The model under review builds one solid part; all positions refer to its coordinate system, in mm. Face numbers are marked on the shaded views. A direction names the side the tool comes from. Coordinates: 2 decimals unless noted, no trailing zeros. Loops run counter-clockwise (first coordinate to the right, second up) from the corner with the lowest first, then second, coordinate; pieces in that order, holes last. Notation, with made-up numbers: (70, 61.5) - (84, 61.5) arc R24 cw to (84, 84.5) - close; hole circle Ø4 at (-37.75, 63.25). An arc over 180 degrees is marked (long way). One line per item, written item: value. Start each with the question number.
1. We need section A-A, the plane x = 0. Give the boundary of the cut face in (y, z).
2. Mouldability with a two-part tool opening along X and no side actions: class the marked faces 4, 5 and 6 as +X half, -X half, draft (parallel to the pull), parting line (faces both ways), or undercut.
3. We need section D-D, the plane y = 0. Give the boundary of the cut face in (x, z).
4. To check wall thickness, follow line 1 (Y direction, x = 0.5, z = -23); line 2 (Z direction, x = -26, y = -8); line 3 (Z direction, x = -22, y = -14.5). State the ranges of each line that lie inside material, in increasing order.
5. Insertion check: P1, Ø13, axis at x = -20.12, z = 9.25, coming from the +Y side; P2, Ø4, axis at x = -20.12, z = 9.25, coming from the -Y side; P3, Ø0.6, axis at y = -17.5, z = 0, coming from the -X side; P4, Ø3, axis at x = -23.5, z = -13.5, coming from the -Y side. Each pin has a flat end and moves straight along its axis. Give the tip position at first contact, or say it passes through.
6. We need section B-B, the plane z = -24.25. Give the boundary of the cut face in (x, y).
7. We need section C-C, the plane x = -14. Give the boundary of the cut face in (y, z).
8. For the marked faces 1, 2 and 3, list the 3-axis set-ups (+Z, -Z, +X, -X, +Y, -Y) from which the entire face can be reached by the end or side of a thin tool; tool diameter is ignored.
from build123d import *

# Parameters (mm, degrees)
F1_DEPTH       = 35
F3_D           = 5
F3_START       = 1.7550021
F3_CBORE_D     = 10
F3_CBORE_DEPTH = 8
F4_W           = 22.4
F4_H           = 2
F5_DEPTH       = 25
F6_R           = 6
F7_DEPTH       = 8


with BuildPart() as f1:
    # F0 (on Top) → F1 (new body, symmetric)
    with BuildSketch(Plane.XY):
        with BuildLine():
            ThreePointArc((-17.3192642082, 2.5086026559), (17.5, 0), (-17.3192642082, -2.5086026559))
            Line((-17.3192642082, -2.5086026559), (-28.1192642082, -2.5086026559))
            Line((-28.1192642082, -2.5086026559), (-28.1192642082, -10.9086026559))
            ThreePointArc((-28.1192642082, -10.9086026559), (-25.7761184577, -16.5654569054), (-20.1192642082, -18.9086026559))
            Line((-20.1192642082, -18.9086026559), (-7.9192642082, -18.9086026559))
            ThreePointArc((-7.9192642082, -18.9086026559), (20.5, 0), (-7.9192642082, 18.9086026559))
            Line((-7.9192642082, 18.9086026559), (-20.1192642082, 18.9086026559))
            ThreePointArc((-20.1192642082, 18.9086026559), (-25.7761184577, 16.5654569054), (-28.1192642082, 10.9086026559))
            Line((-28.1192642082, 10.9086026559), (-28.1192642082, 2.5086026559))
            Line((-28.1192642082, 2.5086026559), (-17.3192642082, 2.5086026559))
        make_face()
    extrude(amount=F1_DEPTH, both=True)

    # F3 (through all)
    # its depths count from where the whole tool has entered the part; down to there all is cleared
    with Locations(Plane.XZ.offset(18.9086026559).offset(-F3_START)):
        with Locations((-20.1192642082, -24.25), (-20.1192642082, -9.25), (-20.1192642082, 9.25), (-20.1192642082, 24.25)):
            CounterBoreHole(F3_D / 2, F3_CBORE_D / 2, F3_CBORE_DEPTH)

    # F4 (on Front) → F5 (cut, symmetric)
    with BuildSketch(Plane.XZ):
        with Locations((-16.9192642082, 0)):
            Rectangle(F4_W, F4_H)
    extrude(amount=F5_DEPTH, both=True, mode=Mode.SUBTRACT)

    # F6 (on Top) → F7 (cut)
    with BuildSketch(Plane.XY):
        with Locations((0, -25)):
            Circle(F6_R)
        with Locations((17.6776695297, -17.6776695297)):
            Circle(F6_R)
        with Locations((25, 0)):
            Circle(F6_R)
        with Locations((17.6776695297, 17.6776695297)):
            Circle(F6_R)
        with Locations((0, 25)):
            Circle(F6_R)
    extrude(amount=-F7_DEPTH, mode=Mode.SUBTRACT)


solid = f1.part
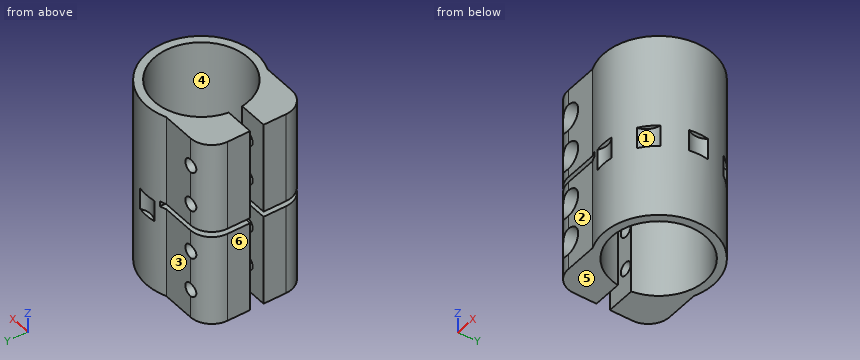
Findings below:
1. outline: (-20.5, -35) - (-17.5, -35) - (-17.5, 35) - (-20.5, 35) - (-20.5, 0) - (-19, 0) - (-19, -8) - (-20.5, -8) - close; (17.5, -35) - (20.5, -35) - (20.5, -8) - (19, -8) - (19, 0) - (20.5, 0) - (20.5, 35) - (17.5, 35) - close
2. face 4: undercut
2. face 5: draft
2. face 6: -X half
3. outline: (17.5, -35) - (20.5, -35) - (20.5, -8) - (19, -8) - (19, 0) - (20.5, 0) - (20.5, 35) - (17.5, 35) - close
4. line 1: -20.49 to -17.49, 17.49 to 20.49
4. line 2: -35 to -1, 1 to 35
4. line 3: -35 to -28.88, -19.62 to -13.88, -4.62 to -1, 1 to 4.62, 13.88 to 19.62, 28.88 to 35
5. P1: y = 18.91
5. P2: through
5. P3: x = -5.72
5. P4: y = -18.67
6. outline: (-28.12, -10.91) arc R8 ccw to (-25.12, -17.15) - (-25.12, -9.15) - (-22.62, -9.15) - (-22.62, -2.51) - (-28.12, -2.51) - close; (-28.12, 2.51) - (-22.62, 2.51) - (-22.62, 18.51) arc R8 ccw to (-28.12, 10.91) - close; (-17.62, -9.15) - (-15.12, -9.15) - (-15.12, -18.91) - (-7.92, -18.91) arc R20.5 ccw (long way) to (-7.92, 18.91) - (-17.62, 18.91) - (-17.62, 2.51) - (-17.32, 2.51) arc R17.5 cw (long way) to (-17.32, -2.51) - (-17.62, -2.51) - close
7. outline: (-18.91, -35) - (-10.5, -35) - (-10.5, -1) - (-18.91, -1) - close; (-18.91, 1) - (-10.5, 1) - (-10.5, 35) - (-18.91, 35) - close; (10.5, -35) - (18.91, -35) - (18.91, -1) - (10.5, -1) - close; (10.5, 1) - (18.91, 1) - (18.91, 35) - (10.5, 35) - close
8. face 1: +X, -Y
8. face 2: +Z, -Z, -X, -Y
8. face 3: +Z, -Z, -X, +Y
